Could you check a few things on this model? Use its own coordinates, in mm. Round coordinates to 2 decimals unless told otherwise and drop trailing zeros. Write each loop counter-clockwise with the first axis right and the second up, starting at its lowest first coordinate (ties: lowest second). Pieces come first, ordered by that corner, then holes. Notation, with made-up numbers: (44, -3.75) -> (100, -3.75) arc R9 cw to (100, 0.25) -> close; hole circle Ø5 at (47.5, 31). An arc over 180 degrees is marked (long way). Answer in a Markdown table with one row per item. Add a question column.
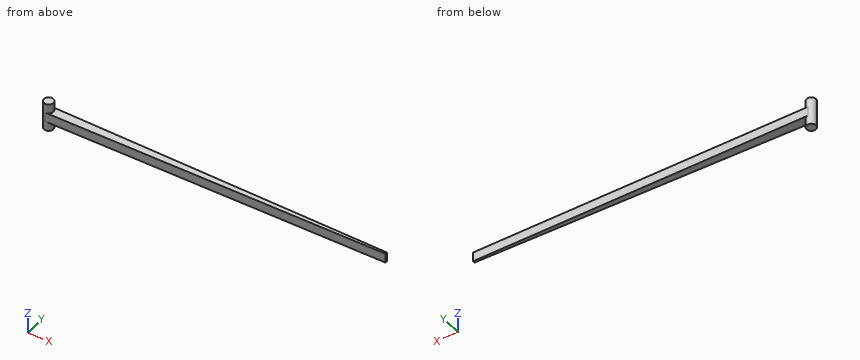
```python
from build123d import *

# Parameters (mm, degrees)
BOSS_EXTRUDE1_DEPTH      = 45
BOSS_EXTRUDE2_DEPTH      = 45
BOSS_EXTRUDE2_DEPTH_BACK = 90
SKETCH2_R                = 22.5


with BuildPart() as part:
    # Sketch1 → Boss-Extrude1 (new body)
    with BuildSketch(Plane.XY):
        Polygon((0, 0), (1600, 0), (1600, -10), (0, -45), align=None)
    extrude(amount=BOSS_EXTRUDE1_DEPTH)

    # Sketch2 → Boss-Extrude2 (add, two sides: drawn at the far end of the back side and taken through both)
    with BuildSketch(Plane.XY.offset(45).offset(-BOSS_EXTRUDE2_DEPTH_BACK)):
        with Locations((0, -22.5)):
            Circle(SKETCH2_R)
    extrude(amount=BOSS_EXTRUDE2_DEPTH + BOSS_EXTRUDE2_DEPTH_BACK)


solid = part.part
```
(1) I need wall thicknesses on L1, parallel to Z at x = 47, y = -6; L2, parallel to X at y = -24.5, z = -32; L3, parallel to X at y = -16, z = -22.5. Which ranges of each line are inside material? Lowest first, please.
(2) Suppose I cut it at D-D, the plane x = 578. Please give me the cut outline in (y, z), then the cut area to 3 significant figures.
(3) Suppose I cut it at B-B, the plane z = -24. Please give me the cut outline in (x, y), then the cut area to 3 significant figures.
(4) Suppose I cut it at C-C, the plane x = 986. Please give me the cut outline in (y, z).
(5) For P1, Ø12, axis at x = 923.5, y = -36, coming from the -Z side; P2, Ø10, axis at y = -5, z = -30, coming from the +X side; P3, Ø1, axis at y = -5.5, z = 70.5, coming from the +X side; P4, Ø8, axis at x = 1099, y = -10.5, coming from the +Z side, each with a flat end and sliding along its axis, tell me the tip position at first contact or that it passes through.
(6) Suppose I cut it at A-A, the plane y = -22.5. Please give me the cut outline in (x, z), then the cut area to 3 significant figures.
Response:
| question | item | result |
|---|---|---|
| 1 | L1 | 0 to 45 |
| 1 | L2 | -22.41 to 22.41 |
| 1 | L3 | -21.54 to 21.54 |
| 2 | outline | (-32.36, 0) -> (0, 0) -> (0, 45) -> (-32.36, 45) -> close |
| 2 | area | 1,460 mm² |
| 3 | outline | circle Ø45 at (0, -22.5) |
| 3 | area | 1,590 mm² |
| 4 | outline | (-23.43, 0) -> (0, 0) -> (0, 45) -> (-23.43, 45) -> close |
| 5 | P1 | through |
| 5 | P2 | x = 18.71 |
| 5 | P3 | x = 15.3 |
| 5 | P4 | z = 45 |
| 6 | outline | (-22.5, -45) -> (22.5, -45) -> (22.5, 0) -> (1028.57, 0) -> (1028.57, 45) -> (22.5, 45) -> (22.5, 90) -> (-22.5, 90) -> close |
| 6 | area | 51,300 mm² |
